from build123d import *

# Parameters (mm, degrees)
EXTRUDE_1_DEPTH = 9
EXTRUDE_2_DEPTH = 3


with BuildPart() as part:
    # 스케치1 → 보스-돌출1 (new, symmetric)
    with BuildSketch(Plane.XY):
        with BuildLine():
            Line((75, -8.660254038), (75, 0))
            Line((75, 0), (65, 0))
            Line((65, 0), (65, -10))
            ThreePointArc((65, -10), (62.656854249, -15.656854249), (57, -18))
            Line((57, -18), (23, -18))
            ThreePointArc((23, -18), (17.343145751, -15.656854249), (15, -10))
            Line((15, -10), (15, 0))
            Line((15, 0), (0, 0))
            Line((0, 0), (0, -22))
            Line((0, -22), (74.105117767, -22))
            Line((74.105117767, -22), (100.176914536, -37.052558883))
            Line((100.176914536, -37.052558883), (106.176914536, -26.660254038))
            Line((106.176914536, -26.660254038), (75, -8.660254038))
        make_face()
    extrude(amount=EXTRUDE_1_DEPTH, both=True)

    # 스케치1<3> → 보스-돌출2 (add, symmetric)
    with BuildSketch(Plane.XY):
        Polygon((80, 0), (75, 0), (75, -8.660254038), (106.176914536, -26.660254038), (111.176914536, -18), align=None)
        with BuildLine():
            Line((65, -10), (65, 0))
            Line((65, 0), (15, 0))
            Line((15, 0), (15, -10))
            ThreePointArc((15, -10), (17.343145751, -15.656854249), (23, -18))
            Line((23, -18), (57, -18))
            ThreePointArc((57, -18), (62.656854249, -15.656854249), (65, -10))
        make_face()
    extrude(amount=EXTRUDE_2_DEPTH, both=True)


solid = part.part
Check sheet for the modelled part. Datum: model origin and axes. Units: mm. A direction names the side the tool comes from. Round coordinates to 2 decimals unless told otherwise and drop trailing zeros. Loops run counter-clockwise (first coordinate to the right, second up) from the corner with the lowest first, then second, coordinate; pieces in that order, holes last. Notation, with made-up numbers: M -31,8 L -5,8 A22 cw -5,25 Z; hole C 77.5,63.5 d1. An arc over 180 degrees is marked long. One line per question, with ' | ' between items. Start each with the question number.
Item 1: Section check C-C (y = -12). Record the boundary of the cut face in (x, z), and give its area (3 significant figures).
Item 2: Set-up check for faces 1 (the face through (15, -5, -6)), 2 (the face through (90.81, -17.79, 6.04)), 3 (the face through (93, -13, -3)): record each of +Z, -Z, +X, -X, +Y, -Y from which the full face is reachable in a straight line by a thin tool's end or side.
Item 3: Scan lines: probe 1 along X at (y, z) = (-3, 4.25); probe 2 along Y at (x, z) = (59, -0.5); probe 3 along Y at (x, z) = (50, 4). Record each from-to range of solid material in increasing order.
Item 4: Release check for a two-part mould opening along X. For faces 4 (the face through (49, -20, -9)), 5 (the face through (65, -5, 6)), 6 (the face through (75, -4, -6)) record: released by +X, released by -X, zero draft, split by the parting line, or undercut.
Item 5: Gauge pin test, flat ends, axial feed: pin 1 Ø6 at (x, z) = (27.5, 2) entering from -Y; pin 2 Ø3 at (y, z) = (-7, -7.5) entering from +X; pin 3 Ø9 at (x, y) = (49.5, -6) entering from -Z. Record the tip position at first contact, or that the pin passes through.
Item 6: Section check A-A (x = 50). Record the boundary of the cut face in (y, z), and give its area (3 significant figures).
Item 7: Section check D-D (y = -16.5). Record the boundary of the cut face in (x, z).
Item 8: Section check B-B (z = -6.25). Record the boundary of the cut face in (x, y).
Worked out:
1) outline: M 0,-9 L 15.25,-9 L 15.25,-3 L 64.75,-3 L 64.75,-9 L 80.78,-9 L 80.78,-3 L 100.78,-3 L 100.78,3 L 80.78,3 L 80.78,9 L 64.75,9 L 64.75,3 L 15.25,3 L 15.25,9 L 0,9 Z | area: 980 mm^2
2) face 1: -Z, +Y | face 2: +Z, +X, +Y | face 3: -Z, +X, +Y
3) probe 1: 0 to 15, 65 to 75 | probe 2: -22 to 0 | probe 3: -22 to -18
4) face 4: zero draft | face 5: undercut | face 6: released by +X
5) pin 1: y = -22 | pin 2: x = 75 | pin 3: z = -3
6) outline: M -22,-9 L -18,-9 L -18,-3 L 0,-3 L 0,3 L -18,3 L -18,9 L -22,9 Z | area: 180 mm^2
7) outline: M 0,-9 L 18.34,-9 L 18.34,-3 L 61.66,-3 L 61.66,-9 L 88.58,-9 L 88.58,-3 L 108.58,-3 L 108.58,3 L 88.58,3 L 88.58,9 L 61.66,9 L 61.66,3 L 18.34,3 L 18.34,9 L 0,9 Z
8) outline: M 0,-22 L 74.11,-22 L 100.18,-37.05 L 106.18,-26.66 L 75,-8.66 L 75,0 L 65,0 L 65,-10 A8 cw 57,-18 L 23,-18 A8 cw 15,-10 L 15,0 L 0,0 Z
